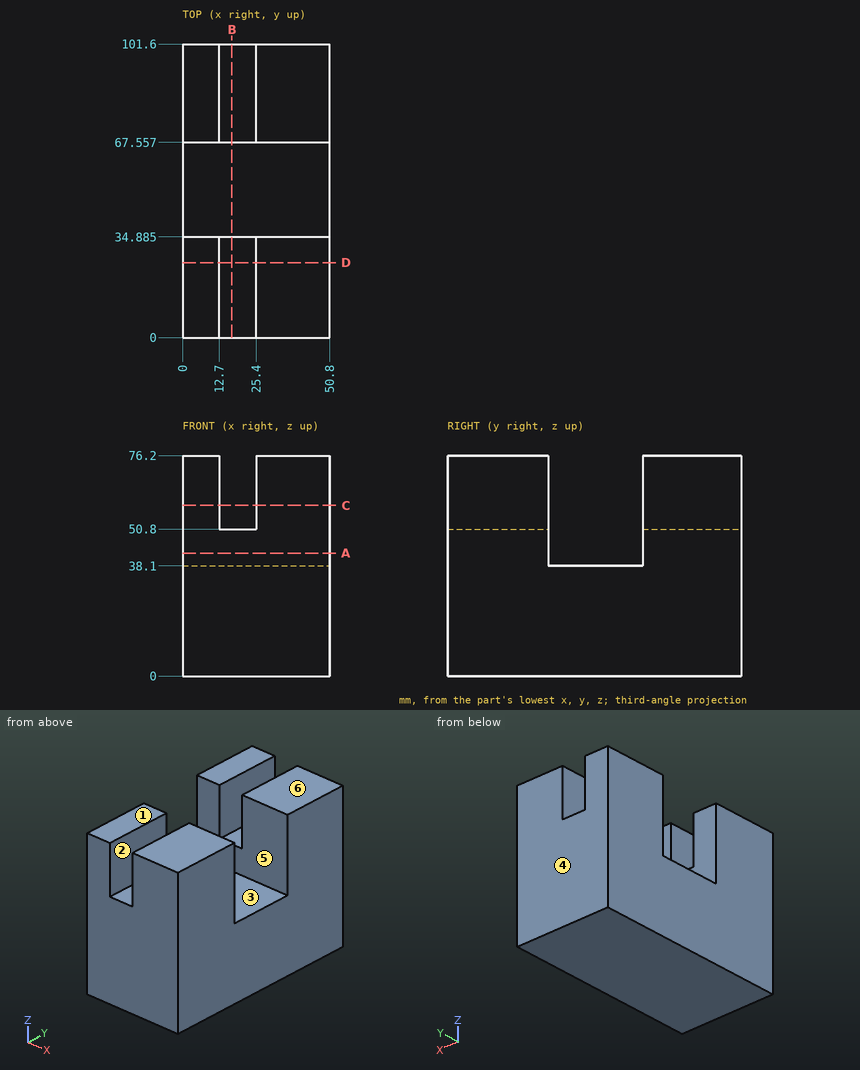
Check sheet for the drawn part. Datum: minimum x, y, z corner. Units: mm. A direction names the side the tool comes from. Give positions to 0.01 mm unless a question says otherwise; leave off trailing zeros. Order: outer loops, then holes, each group sorted by start corner. A loop starts at its lowest first (then second) coordinate and runs counter-clockwise, first axis right, second up. Notation, with made-up numbers: (-7.5, 11) -> (3.5, 11) arc R24 cw to (3.5, 25) -> close; hole circle Ø4 at (5, 24.5). An arc over 180 degrees is marked (long way). Use a Markdown table: item, result.
1) Tool access check on the marked faces 1, 2 and 3. Record the directions out of +Z, -Z, +X, -X, +Y, -Y that give a thin tool (end or side, any length) a straight path to the whole face; none if there is none.
Results:
| item | result |
|---|---|
| face 1 | +Z, +X, -X, +Y, -Y |
| face 2 | +Z, +Y, -Y |
| face 3 | +Z, +X, -X |
2) Section check D-D, the plane y = 26. Record the boundary of the cut face in (x, z), then the cut area to 3 significant figures.
Results:
| item | result |
|---|---|
| outline | (0, 0) -> (50.8, 0) -> (50.8, 76.2) -> (25.4, 76.2) -> (25.4, 50.8) -> (12.7, 50.8) -> (12.7, 76.2) -> (0, 76.2) -> close |
| area | 3,550 mm² |
3) Depth check by flat-ended pin: pin 1 Ø1 at (x, y) = (8, 39) entering from +Z; pin 2 Ø6.5 at (x, y) = (22, 79) entering from +Z. Enter the tip coordinate at first touch or a pass-through.
Results:
| item | result |
|---|---|
| pin 1 | z = 38.1 |
| pin 2 | z = 50.8 |
4) Section check C-C, the plane z = 59. Record the boundary of the cut face in (x, y) (1 decimal), then the cut area to 3 significant figures.
Results:
| item | result |
|---|---|
| outline | (0, 0) -> (12.7, 0) -> (12.7, 34.9) -> (0, 34.9) -> close; (0, 67.6) -> (12.7, 67.6) -> (12.7, 101.6) -> (0, 101.6) -> close; (25.4, 0) -> (50.8, 0) -> (50.8, 34.9) -> (25.4, 34.9) -> close; (25.4, 67.6) -> (50.8, 67.6) -> (50.8, 101.6) -> (25.4, 101.6) -> close |
| area | 2,630 mm² |
5) Mould release check, pull along Y, two halves, no side actions. Record for the marked faces 4, 5 and 6: pulls with the +Y half, pulls with the -Y half, needs draft (parallel to the pull), parting line crosses it, or undercut.
Results:
| item | result |
|---|---|
| face 4 | pulls with the +Y half |
| face 5 | undercut |
| face 6 | needs draft |
6) Material ranges on probe 1 along Y at (x, z) = (37.5, 50) (1 decimal); probe 2 along X at (y, z) = (97.5, 69.5); probe 3 along Z at (x, y) = (19, 16), recorded low to high.
Results:
| item | result |
|---|---|
| probe 1 | 0 to 34.9, 67.6 to 101.6 |
| probe 2 | 0 to 12.7, 25.4 to 50.8 |
| probe 3 | 0 to 50.8 |
7) Section check B-B, the plane x = 17. Record the boundary of the cut face in (y, z) (1 decimal).
Results:
| item | result |
|---|---|
| outline | (0, 0) -> (101.6, 0) -> (101.6, 50.8) -> (67.6, 50.8) -> (67.6, 38.1) -> (34.9, 38.1) -> (34.9, 50.8) -> (0, 50.8) -> close |
8) Section check A-A, the plane z = 42.5. Record the boundary of the cut face in (x, y) (1 decimal), then the cut area to 3 significant figures.
Results:
| item | result |
|---|---|
| outline | (0, 0) -> (50.8, 0) -> (50.8, 34.9) -> (0, 34.9) -> close; (0, 67.6) -> (50.8, 67.6) -> (50.8, 101.6) -> (0, 101.6) -> close |
| area | 3,500 mm² |
